Autodesk Inventor part; units mm, degrees
ref_plane "YZ Plane" through (0, 0, 0) normal (1, 0, 0) x (0, 1, 0)
ref_plane "XZ Plane" through (0, 0, 0) normal (0, 1, 0) x (-1, 0, 0)
ref_plane "XY Plane" through (0, 0, 0) normal (0, 0, 1) x (1, 0, 0)
sketch "Sketch1" plane through (0, 0, 0) normal (0, 0, 1) x (1, 0, 0)
  line L0 (0, 0) -> (14.986, 0)
  line L1 (14.986, 0) -> (14.986, 5.588)
  line L2 (14.986, 5.588) -> (0, 5.588)
  line L3 (0, 5.588) -> (0, 0)
  line L4 (0, 5.588) -> (19.05, 5.588)
  line L5 (19.05, 5.588) -> (19.05, 9.525)
  line L6 (15.875, 12.7) -> (0, 12.7)
  line L7 (0, 12.7) -> (0, 5.588)
  arc A0 (19.05, 9.525) -> (15.875, 12.7) centre (15.875, 9.525) ccw
  dimension "d0" = 14.986
  dimension "d1" = 5.588
  dimension "d2" = 19.05
  dimension "d3" = 12.7
  dimension "d4" = 3.175
revolve "Revolution1" add sketch "Sketch1" angle 360 about axis through (0, 5.588, 0) along (0, -1, 0)
chamfer "Chamfer1" distance 1.5875 angle 45 1 edges at (-14.986, 0, 0)
properties part number "2016.06.09 Judson M204 bung cover"
Build history of the part. All positions in model axes, mm. A direction names the side the tool comes from. Round coordinates to 2 decimals unless told otherwise and drop trailing zeros. Write each loop counter-clockwise with the first axis right and the second up, starting at its lowest first coordinate (ties: lowest second). Pieces come first, ordered by that corner, then holes. Notation, with made-up numbers: (24.5, 80.25) - (71.5, 80.25) arc R30 ccw to (71.5, 116.25) - close; hole circle Ø8 at (35.5, 83). An arc over 180 degrees is marked (long way). Write each question's results on one line, items separated by ' | '. Start each with the question number.
Item 1: Wall check: L1, parallel to Y at x = 15.5, z = 1; L2, parallel to Z at x = 5, y = 7; L3, parallel to X at y = 11.75, z = 15. Give the ranges that are in metal, low to high. Write a range as [from, to].
Item 2: Saw through at C-C (y = 3). Write the cut outline in (x, z), and give its area (3 significant figures).
Item 3: Drop flat-ended pins along their axis: P1, Ø3, axis at x = -2.5, y = 9.5, coming from the -Z side; P2, Ø4, axis at x = 7, z = -12.5, coming from the -Y side; P3, Ø1.5, axis at x = 4.5, y = 4, coming from the -Z side; P4, Ø2, axis at x = -7.5, y = 9.5, coming from the -Z side. Give the stop position or say it passes through.
Item 4: Saw through at D-D (y = 8.75). Write the cut outline in (x, z).
Item 5: Which spindle directions (+Z, -Z, +X, -X, +Y, -Y) get a long thin tool onto all of the face, cutting with end or side? Do faces 1 (the face through (0, 0, 0)), 2 (the face through (8, 5.588, -13)). Say none if no direction does.
Results are:
1) L1: y = [5.59, 12.7] | L2: z = [-18.38, 18.38] | L3: x = [-10.2, 10.2]
2) outline: circle Ø29.97 at (0, 0) | area: 706 mm²
3) P1: stops at z = -19.02 | P2: stops at y = 0 | P3: stops at z = -14.51 | P4: stops at z = -17.91
4) outline: circle Ø38.1 at (0, 0)
5) face 1: +Z, -Z, +X, -X, -Y | face 2: -Y
